Drawing for the job (mm, zero at the part's lowest x, y, z). Round coordinates to 2 decimals unless told otherwise and drop trailing zeros. Write each loop counter-clockwise with the first axis right and the second up, starting at its lowest first coordinate (ties: lowest second). Pieces come first, ordered by that corner, then holes. Notation, with made-up numbers: M 16,-7 L 65,-7 A15 ccw 65,21 Z; hole C 63.5,-21.5 d4. An arc over 180 degrees is marked long. Use a Markdown table: item, result.
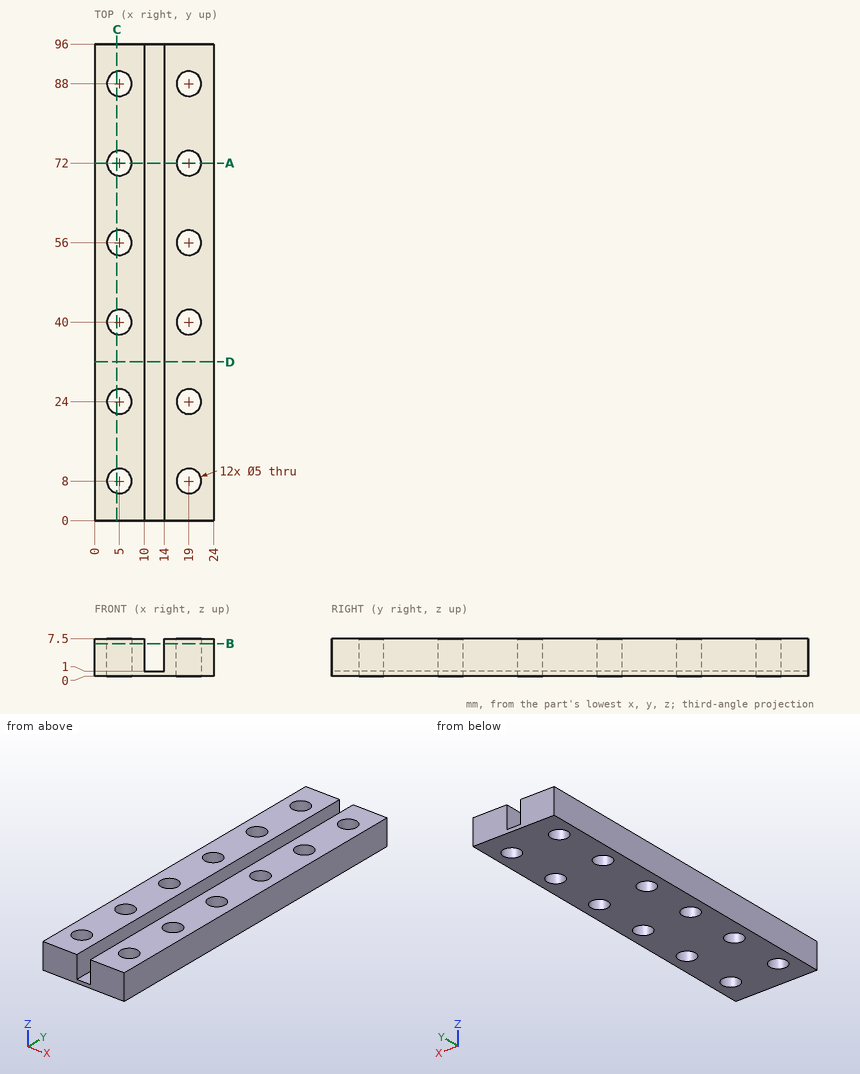
Q1. Cut at C-C on x = 4.5. Give the cut face in (y, z), and give its area (3 significant figures).
Response values:
| item | result |
|---|---|
| outline | M 0,0 L 5.55,0 L 5.55,7.5 L 0,7.5 Z; M 10.45,0 L 21.55,0 L 21.55,7.5 L 10.45,7.5 Z; M 26.45,0 L 37.55,0 L 37.55,7.5 L 26.45,7.5 Z; M 42.45,0 L 53.55,0 L 53.55,7.5 L 42.45,7.5 Z; M 58.45,0 L 69.55,0 L 69.55,7.5 L 58.45,7.5 Z; M 74.45,0 L 85.55,0 L 85.55,7.5 L 74.45,7.5 Z; M 90.45,0 L 96,0 L 96,7.5 L 90.45,7.5 Z |
| area | 500 mm2 |
Q2. Drill centre lines: L1, parallel to X at y = 45, z = 3; L2, parallel to X at y = 7, z = 4.75; L3, parallel to X at y = 10, z = 0.75. Where is each one in solid material? Low to high.
Response values:
| item | result |
|---|---|
| L1 | x = 0 to 10, 14 to 24 |
| L2 | x = 0 to 2.71, 7.29 to 10, 14 to 16.71, 21.29 to 24 |
| L3 | x = 0 to 3.5, 6.5 to 17.5, 20.5 to 24 |
Q3. Cut at D-D on y = 32. Give the cut face in (x, z).
Response values:
| item | result |
|---|---|
| outline | M 0,0 L 24,0 L 24,7.5 L 14,7.5 L 14,1 L 10,1 L 10,7.5 L 0,7.5 Z |
Q4. Cut at A-A on y = 72. Give the cut face in (x, z), and give its area (3 significant figures).
Response values:
| item | result |
|---|---|
| outline | M 0,0 L 2.5,0 L 2.5,7.5 L 0,7.5 Z; M 7.5,0 L 16.5,0 L 16.5,7.5 L 14,7.5 L 14,1 L 10,1 L 10,7.5 L 7.5,7.5 Z; M 21.5,0 L 24,0 L 24,7.5 L 21.5,7.5 Z |
| area | 79.0 mm2 |
Q5. Cut at B-B on z = 6.5. Count the separate pieces of the cut face and the enclosed holes in it, and give its area (3 significant figures).
Response values:
| item | result |
|---|---|
| separate pieces | 2 |
| enclosed holes | 12 |
| area | 1,680 mm2 |
